Check sheet for the drawn part. Datum: minimum x, y, z corner. Units: mm. A direction names the side the tool comes from. Coordinates: 2 decimals unless noted, no trailing zeros. Loops run counter-clockwise (first coordinate to the right, second up) from the corner with the lowest first, then second, coordinate; pieces in that order, holes last.
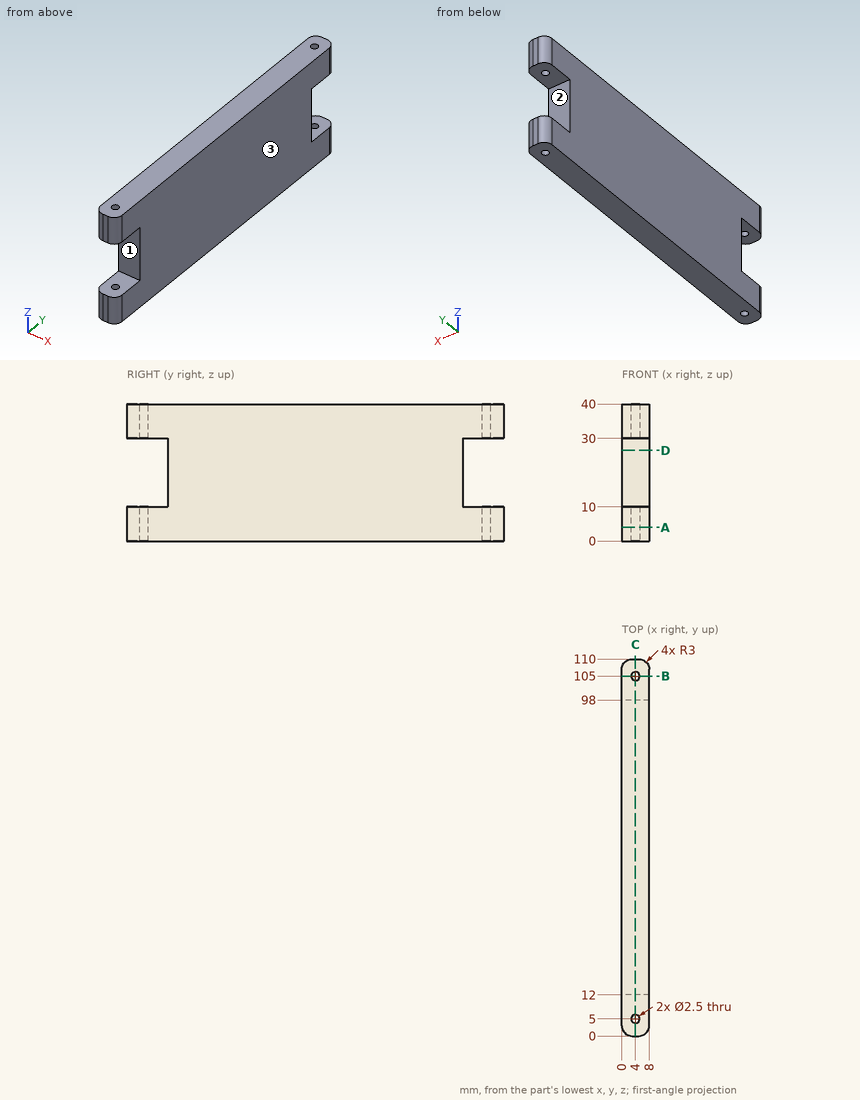
(1) Sectioned sample at A-A on z = 4. Record the cut outline in (x, y).
Findings:
outline: (0, 3) arc R3 ccw to (3, 0) - (5, 0) arc R3 ccw to (8, 3) - (8, 107) arc R3 ccw to (5, 110) - (3, 110) arc R3 ccw to (0, 107) - close; hole circle Ø2.5 at (4, 5); hole circle Ø2.5 at (4, 105)
(2) Sectioned sample at C-C on x = 4. Record the cut outline in (y, z).
Findings:
outline: (0, 0) - (3.75, 0) - (3.75, 10) - (0, 10) - close; (0, 30) - (3.75, 30) - (3.75, 40) - (0, 40) - close; (6.25, 0) - (103.75, 0) - (103.75, 10) - (98, 10) - (98, 30) - (103.75, 30) - (103.75, 40) - (6.25, 40) - (6.25, 30) - (12, 30) - (12, 10) - (6.25, 10) - close; (106.25, 0) - (110, 0) - (110, 10) - (106.25, 10) - close; (106.25, 30) - (110, 30) - (110, 40) - (106.25, 40) - close
(3) Scan lines: L1, parallel to Y at x = 4, z = 3; L2, parallel to X at y = 105, z = 2; L3, parallel to Z at x = 7.5, y = 105.5. Record each from-to range of solid material in increasing order.
Findings:
L1: y = 0 to 3.75, 6.25 to 103.75, 106.25 to 110
L2: x = 0 to 2.75, 5.25 to 8
L3: z = 0 to 10, 30 to 40
(4) Sectioned sample at D-D on z = 26.5. Record the cut outline in (x, y).
Findings:
outline: (0, 12) - (8, 12) - (8, 98) - (0, 98) - close
(5) Sectioned sample at B-B on y = 105. Record the cut outline in (x, z).
Findings:
outline: (0, 0) - (2.75, 0) - (2.75, 10) - (0, 10) - close; (0, 30) - (2.75, 30) - (2.75, 40) - (0, 40) - close; (5.25, 0) - (8, 0) - (8, 10) - (5.25, 10) - close; (5.25, 30) - (8, 30) - (8, 40) - (5.25, 40) - close
(6) Gauge pin test, flat ends, axial feed: pin 1 Ø2 at (x, y) = (4, 105) entering from -Z; pin 2 Ø4 at (x, y) = (4, 5) entering from +Z; pin 3 Ø2 at (x, z) = (2, 23.5) entering from -Y; pin 4 Ø4 at (x, z) = (1.5, 24.5) entering from +Y. Record the tip position at first contact, or that the pin passes through.
Findings:
pin 1: passes through
pin 2: stops at z = 40
pin 3: stops at y = 12
pin 4: stops at y = 98
(7) Access from +Z, -Z, +X, -X, +Y, -Y to the whole of each face (thin tool, end or side, straight path). Record for the marked faces 1, 2 and 3.
Findings:
face 1: +X, -X, -Y
face 2: +X, -X, +Y
face 3: +Z, -Z, +X, +Y, -Y
